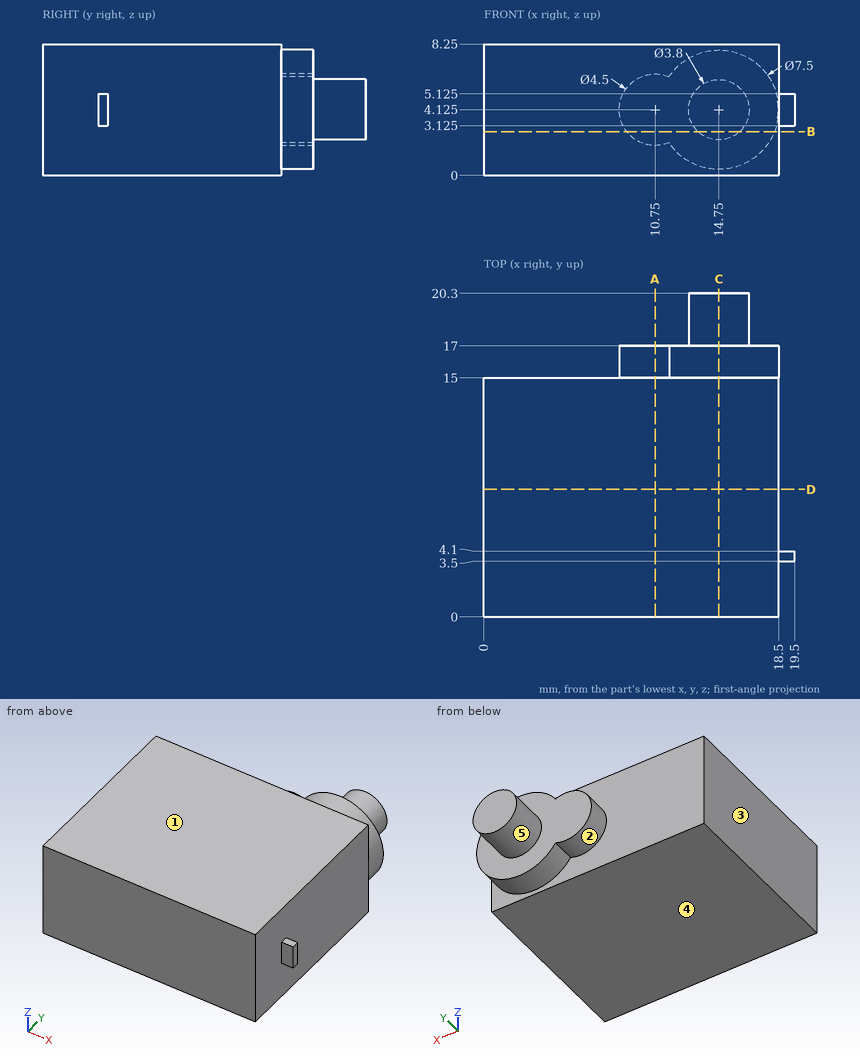
Answer from the drawing. Dimensions are ordinates in mm from the lowest x, y and z of the part. A direction names the side the tool comes from. Round coordinates to 2 decimals unless told otherwise and drop trailing zeros. Write each loop counter-clockwise with the first axis right and the second up, starting at its lowest first coordinate (ties: lowest second). Pieces come first, ordered by that corner, then holes. Notation, with made-up numbers: M -3,50.25 L 41,50.25 A23 cw 41,65.25 Z; hole C 13.25,44.5 d1. An arc over 180 degrees is marked long. Write each question's results on one line, items separated by ' | '. Start each with the question number.
Item 1: Find section A-A on x = 10.75. Write down the section's boundary in (y, z) (3 decimals).
Item 2: Which of the six approach directions +Z, -Z, +X, -X, +Y, -Y give full straight-line access (tool end or side, diameter ignored) to the marked faces 4 and 5?
Item 3: Given pin 1 Ø0.5 at (x, y) = (19, 4) entering from +Z (3 decimals); pin 2 Ø2.5 at (y, z) = (6, 4) entering from +X; pin 3 Ø0.5 at (x, z) = (19, 4.5) entering from +Y, each flat-ended and moving along its own axis, determine where each tip first touches the part or whether it passes through.
Item 4: Find section C-C on x = 14.75. Write down the section's boundary in (y, z) (3 decimals).
Item 5: Find section D-D on y = 8. Write down the section's boundary in (x, z).
Item 6: The mould has two halves that part along X. Classify the marked faces 1, 2 and 3: +X half, -X half, draft (parallel to the pull), parting line (faces both ways), or undercut.
Item 7: Straight lines are drawn through the part: probe 1 along X at (y, z) = (2.5, 2); probe 2 along Y at (x, z) = (8, 2.5); probe 3 along Y at (x, z) = (10.5, 3). For each, find the intervals that lie inside material, in ascending order.
Item 8: Find section B-B on z = 2.75. Write down the section's boundary in (x, y), and give its area (3 significant figures).
Answer block:
1) outline: M 0,0 L 15,0 L 15,1.875 L 17,1.875 L 17,6.375 L 15,6.375 L 15,8.25 L 0,8.25 Z
2) face 4: -Z, +X, -X, +Y, -Y | face 5: +Y
3) pin 1: stops at z = 5.125 | pin 2: stops at x = 18.5 | pin 3: stops at y = 4.1
4) outline: M 0,0 L 15,0 L 15,0.375 L 17,0.375 L 17,2.225 L 20.3,2.225 L 20.3,6.025 L 17,6.025 L 17,7.875 L 15,7.875 L 15,8.25 L 0,8.25 Z
5) outline: M 0,0 L 18.5,0 L 18.5,8.25 L 0,8.25 Z
6) face 1: draft | face 2: undercut | face 3: -X half
7) probe 1: x = 0 to 18.5 | probe 2: y = 0 to 15 | probe 3: y = 0 to 17
8) outline: M 0,0 L 18.5,0 L 18.5,15 L 18.24,15 L 18.24,17 L 16.06,17 L 16.06,20.3 L 13.44,20.3 L 13.44,17 L 8.97,17 L 8.97,15 L 0,15 Z | area: 305 mm²
